Autodesk Inventor part; units mm, degrees
ref_plane "YZ Plane" through (0, 0, 0) normal (1, 0, 0) x (0, 1, 0)
ref_plane "XZ Plane" through (0, 0, 0) normal (0, 1, 0) x (-1, 0, 0)
ref_plane "XY Plane" through (0, 0, 0) normal (0, 0, 1) x (1, 0, 0)
sketch "Sketch1" plane through (0, 0, 0) normal (0, 1, 0) x (-1, 0, 0)
  line L0 (0, 0) -> (0, -16)
  line L1 (0, -16) -> (4, -16)
  line L2 (0, 0) -> (4, 0)
  line L3 (4, 0) -> (4, -6.5)
  line L4 (4, -16) -> (4, -13)
  line L5 (4, -13) -> (7, -13)
  line L6 (7, -13) -> (7, -4.5)
  line L7 (7, -4.5) -> (4, -6.5)
  dimension "d0" = 16
  dimension "d1" = 4
  dimension "d2" = 6.5
  dimension "d3" = 3
  dimension "d4" = 3
  dimension "d5" = 8.5
extrude "Extrusion1" add sketch "Sketch1" along normal blind 32
sketch "Sketch2" plane through (-7, 0, -13) normal (-1, 0, 0) x (0, 0, 1)
  line L0 (0, 0) -> (8.5, 0)
  line L1 (8.5, 0) -> (8.5, 32)
  line L2 (0, 32) -> (8.5, 32)
  line L3 (0, 0) -> (0, 32)
  line L4 (0, 32) -> (8.5, 32)
  line L5 (5.5, 32) -> (5.5, 7)
  line L6 (5.5, 7) -> (0, 7)
  line L7 (0, 0) -> (0, 32)
  point P0 (13, 0)
  dimension "d8" = 25
  dimension "d9" = 5.5
extrude "Extrusion2" cut sketch "Sketch2" against normal blind 3 contours L3 L2 L5 L6
sketch "Sketch3" plane through (-4, 0, -16) normal (-1, 0, 0) x (0, 0, 1)
  line L0 (0, 0) -> (3, 0)
  line L1 (3, 0) -> (3, 7)
  line L2 (8.5, 7) -> (3, 7)
  line L3 (8.5, 32) -> (8.5, 7)
  line L4 (0, 32) -> (8.5, 32)
  line L5 (0, 0) -> (0, 32)
  line L6 (0, 0) -> (0, 32)
  line L7 (0, 32) -> (0, 20)
  line L8 (0, 20) -> (3, 20)
  line L9 (8.5, 32) -> (8.5, 7)
  line L10 (0, 32) -> (8.5, 32)
  line L11 (3, 32) -> (3, 17)
  line L12 (3, 17) -> (8.5, 17)
  line L13 (0, 0) -> (0, 32)
  line L14 (0, 7) -> (3, 7)
  point P0 (16, 0)
  dimension "d12" = 12
  dimension "d13" = 15
  dimension "d14" = 3
extrude "Extrusion3" cut sketch "Sketch3" against normal blind 4 contours L5 L8 L11 L12 L3 L2 L14
properties part number "Inner Rails 2"
Geometry check sheet. Reference: the model listing, model coordinates, mm. A direction names the side the tool comes from. Coordinates: 2 decimals unless noted, no trailing zeros. Order: outer loops, then holes, each group sorted by start corner. A loop starts at its lowest first (then second) coordinate and runs counter-clockwise, first axis right, second up. Notation, with made-up numbers: (33, -24) - (49, -24) arc R17 ccw to (49, 8) - close; hole circle Ø6 at (64.5, 75.5). An arc over 180 degrees is marked (long way). Answer in a Markdown table with one row per item. Add a question column.
1. Section check A-A (z = -14.25). Enter the section's corners in (x, y), plus the area to 3 significant figures.
2. Access from +Z, -Z, +X, -X, +Y, -Y to the whole of each face (thin tool, end or side, straight path). Record for faces 5 (the face through (-4, 16, -3)), 6 (the face through (-2, 17, -10)), 7 (the face through (-4, 3, -15)), 8 (the face through (-4, 24, -12)).
3. Section check B-B (x = -0.5). Enter the section's corners in (y, z).
4. Draft check along Y on faces 1 (the face through (-3, 0, -8)), 2 (the face through (0, 16, -6)), 3 (the face through (-4.3, 16.9, -7.5)), 4 (the face through (-2, 32, -8)). Enter one of: +Y half, -Y half, draft (parallel to the pull), parting line (faces both ways), or undercut.
5. Section check C-C (y = 29). Enter the section's corners in (x, z), plus the area to 3 significant figures.
6. Section check D-D (z = -10). Enter the section's corners in (x, y), plus the area to 3 significant figures.
7. Gauge pin test, flat ends, axial feed: pin 1 Ø3.5 at (y, z) = (4, -14) entering from -X; pin 2 Ø1.5 at (x, y) = (-5.5, 4.5) entering from -Z; pin 3 Ø9.5 at (y, z) = (21.5, -13.5) entering from -X. Record the tip position at first contact, or that the pin passes through.
8. Material ranges on L1, parallel to Y at x = -2.75, z = -10.5; L2, parallel to Y at x = -3, z = -14.5; L3, parallel to Z at x = -3, y = 18, recorded low to high. Write a range as [from, to].
Data:
| question | item | result |
|---|---|---|
| 1 | outline | (-4, 0) - (0, 0) - (0, 7) - (-4, 7) - close; (-4, 20) - (0, 20) - (0, 32) - (-4, 32) - close |
| 1 | area | 76.0 mm² |
| 2 | face 5 | +Z, +Y, -Y |
| 2 | face 6 | -Z, +X, -X |
| 2 | face 7 | -Z, -X, +Y, -Y |
| 2 | face 8 | -Z, -X, +Y |
| 3 | outline | (0, -16) - (7, -16) - (7, -7.5) - (17, -7.5) - (17, -13) - (20, -13) - (20, -16) - (32, -16) - (32, 0) - (0, 0) - close |
| 4 | face 1 | -Y half |
| 4 | face 2 | draft |
| 4 | face 3 | undercut |
| 4 | face 4 | +Y half |
| 5 | outline | (-7, -7.5) - (-4, -7.5) - (-4, -16) - (0, -16) - (0, 0) - (-4, 0) - (-4, -6.5) - (-7, -4.5) - close |
| 5 | area | 70.0 mm² |
| 6 | outline | (-7, 0) - (0, 0) - (0, 7) - (-7, 7) - close; (-4, 17) - (0, 17) - (0, 32) - (-4, 32) - close |
| 6 | area | 109 mm² |
| 7 | pin 1 | stops at x = -7 |
| 7 | pin 2 | stops at z = -13 |
| 7 | pin 3 | stops at x = -4 |
| 8 | L1 | y = [0, 7], [17, 32] |
| 8 | L2 | y = [0, 7], [20, 32] |
| 8 | L3 | z = [-13, 0] |
